Source: three-view drawing plus pictorial views. Frame: mm from the lowest corner of the part. A direction names the side the tool comes from. Give positions to 0.01 mm unless a question says otherwise; leave off trailing zeros. Loops run counter-clockwise (first coordinate to the right, second up) from the corner with the lowest first, then second, coordinate; pieces in that order, holes last. Notation, with made-up numbers: M -24,-37.5 L 31,-37.5 A10 ccw 31,-22.5 Z; hole C -3,57.25 d1. An arc over 180 degrees is marked long. Put each result on its own line as item: value. Start each with the question number.
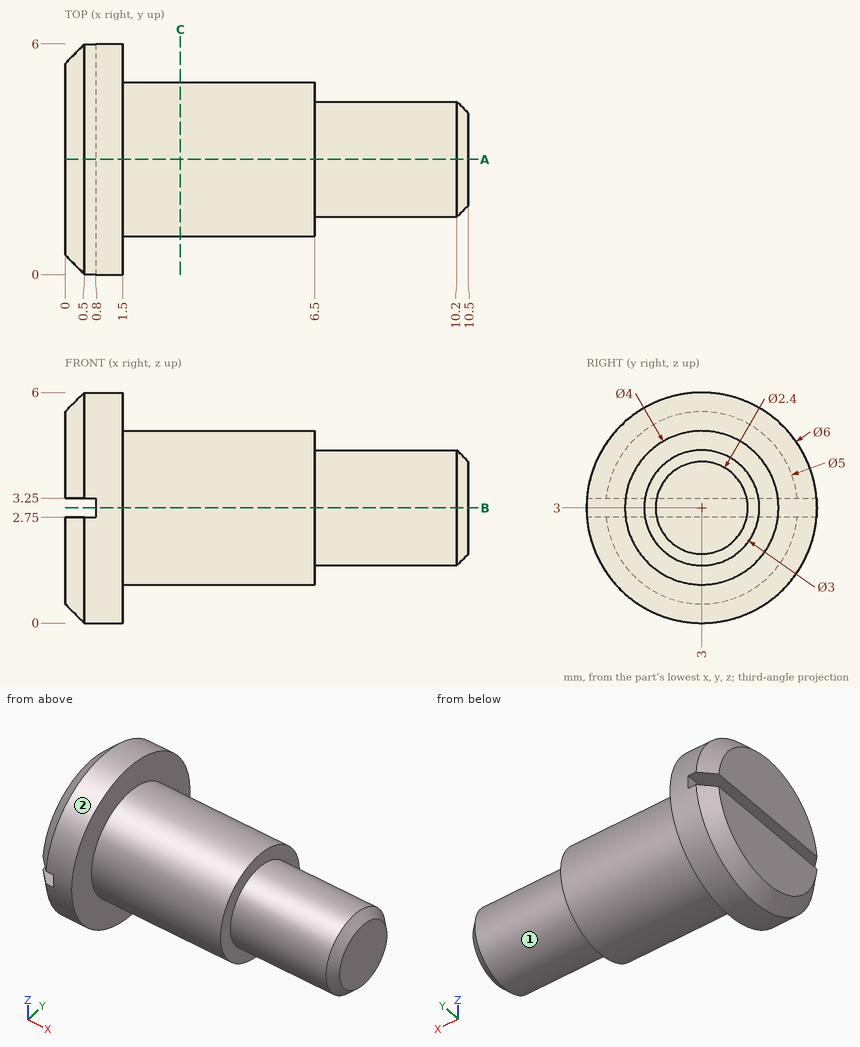
1. Section B-B, the plane z = 3. Output: boundary loops of the cut face in (x, y), plus the area to 3 significant figures.
2. Section A-A, the plane y = 3. Output: boundary loops of the cut face in (x, z).
3. Set-up query: the marked faces 1 and 2. Return all of +Z, -Z, +X, -X, +Y, -Y with unobstructed straight access to the full face (end or side cutting, diameter ignored); none if empty.
4. Section C-C, the plane x = 3. Output: boundary loops of the cut face in (y, z), plus the area to 3 significant figures.
5. Contact query for flat-ended pins moving along their axis: pin 1 (1.5 mm diameter, centred on x = 8.5, z = 2, fed in from +Y); pin 2 (3 mm diameter, centred on y = 1.5, z = 3.5, fed in from +X); pin 3 (3 mm diameter, centred on x = 1.5, y = 5.5, fed in from +Z). Output: stop coordinate, or through.
6. Ray query, line 1 (X direction, y = 4.55, z = 4.6); line 2 (Z direction, x = 8, y = 3.1); line 3 (X direction, y = 3.85, z = 3.1). Return the intervals inside material, ascending.
Results found:
1. outline: M 0.8,0 L 1.5,0 L 1.5,1 L 6.5,1 L 6.5,1.5 L 10.2,1.5 L 10.5,1.8 L 10.5,4.2 L 10.2,4.5 L 6.5,4.5 L 6.5,5 L 1.5,5 L 1.5,6 L 0.8,6 Z
1. area: 36.1 mm²
2. outline: M 0,0.5 L 0.5,0 L 1.5,0 L 1.5,1 L 6.5,1 L 6.5,1.5 L 10.2,1.5 L 10.5,1.8 L 10.5,4.2 L 10.2,4.5 L 6.5,4.5 L 6.5,5 L 1.5,5 L 1.5,6 L 0.5,6 L 0,5.5 L 0,3.25 L 0.8,3.25 L 0.8,2.75 L 0,2.75 Z
3. face 1: +X
3. face 2: +X, -X
4. outline: C 3,3 d4
4. area: 12.6 mm²
5. pin 1: y = 4.48
5. pin 2: x = 10.5
5. pin 3: z = 5.83
6. line 1: 0 to 1.5
6. line 2: 1.5 to 4.5
6. line 3: 0.8 to 10.5
